Geometry: see drawing. Coordinates: mm, zero at the bounding-box minimum. A direction names the side the tool comes from. Round coordinates to 2 decimals unless told otherwise and drop trailing zeros. Loops run counter-clockwise (first coordinate to the right, second up) from the corner with the lowest first, then second, coordinate; pieces in that order, holes last. Notation, with made-up numbers: M 39.25,-39.5 L 56.25,-39.5 A26 cw 56.25,-11.5 Z; hole C 59,76.25 d5. An arc over 180 degrees is marked long. Answer as a JSON object with one key per item and string values.
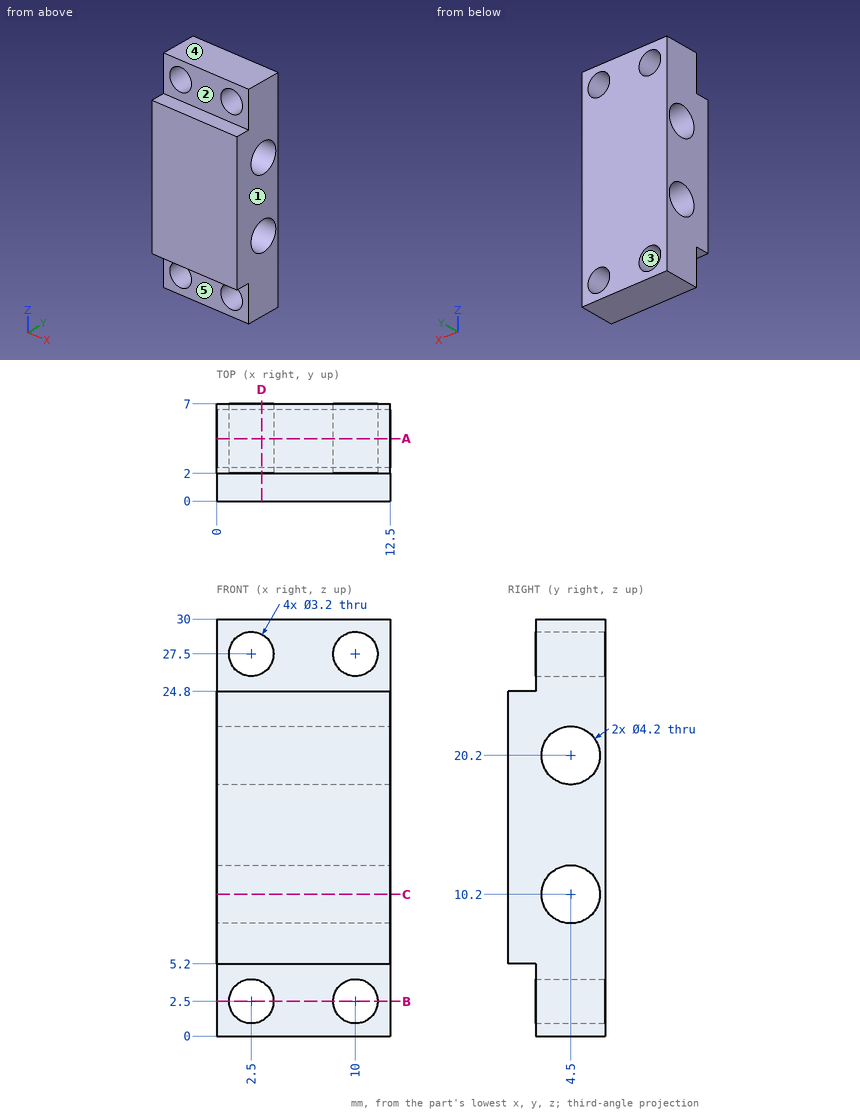
1) Section query D-D (x = 3.25). Return the cut outline in (y, z), and give its area (3 significant figures).
Results:
{"outline": "M 0,5.2 L 2,5.2 L 2,3.91 L 7,3.91 L 7,26.09 L 2,26.09 L 2,24.8 L 0,24.8 Z; M 2,0 L 7,0 L 7,1.09 L 2,1.09 Z; M 2,28.91 L 7,28.91 L 7,30 L 2,30 Z; hole C 4.5,10.2 d4.2; hole C 4.5,20.2 d4.2", "area": "133 mm2"}
2) Reachability of the marked faces 4 and 5 from +Z, -Z, +X, -X, +Y, -Y: full face, straight path, thin tool, end or side. Return the list, or none.
Results:
{"face 4": "+Z, +X, -X, +Y, -Y", "face 5": "-Z, +X, -X, -Y"}
3) Pull-direction query (X, two-part tool) for the marked faces 1, 2 and 3; classes: +X half, -X half, draft (parallel to the pull), parting line (faces both ways), or undercut.
Results:
{"face 1": "+X half", "face 2": "draft", "face 3": "undercut"}
4) Pin query (flat end, axial travel): P1, Ø2.5, axis at y = 4.5, z = 20.2, coming from the -X side; P2, Ø5.5, axis at x = 5.5, z = 28, coming from the -Y side; P3, Ø1.6, axis at x = 7.5, y = 0.5, coming from the -Z side; P4, Ø1, axis at x = 5, y = 1, coming from the +Z side. Return the tip coordinate at first contact, or that it passes through.
Results:
{"P1": "through", "P2": "y = 2", "P3": "z = 5.2", "P4": "z = 24.8"}
5) Section query A-A (y = 4.5). Return the cut outline in (x, z), and give its area (3 significant figures).
Results:
{"outline": "M 0,0 L 12.5,0 L 12.5,8.1 L 0,8.1 Z; M 0,12.3 L 12.5,12.3 L 12.5,18.1 L 0,18.1 Z; M 0,22.3 L 12.5,22.3 L 12.5,30 L 0,30 Z; hole C 2.5,2.5 d3.2; hole C 2.5,27.5 d3.2; hole C 10,2.5 d3.2; hole C 10,27.5 d3.2", "area": "238 mm2"}
6) Section query C-C (z = 10.2). Return the cut outline in (x, y), and give its area (3 significant figures).
Results:
{"outline": "M 0,0 L 12.5,0 L 12.5,2.4 L 0,2.4 Z; M 0,6.6 L 12.5,6.6 L 12.5,7 L 0,7 Z", "area": "35.0 mm2"}
7) Section query B-B (z = 2.5). Return the cut outline in (x, y).
Results:
{"outline": "M 0,2 L 0.9,2 L 0.9,7 L 0,7 Z; M 4.1,2 L 8.4,2 L 8.4,7 L 4.1,7 Z; M 11.6,2 L 12.5,2 L 12.5,7 L 11.6,7 Z"}
8) Ray query, line 1 (Z direction, x = 10, y = 4.4); line 2 (X direction, y = 3.75, z = 2.5); line 3 (X direction, y = 3.5, z = 3). Return the intervals inside material, ascending.
Results:
{"line 1": "0 to 0.9, 4.1 to 8.1, 12.3 to 18.1, 22.3 to 25.9, 29.1 to 30", "line 2": "0 to 0.9, 4.1 to 8.4, 11.6 to 12.5", "line 3": "0 to 0.98, 4.02 to 8.48, 11.52 to 12.5"}
